Design review of the part built by this model. Coordinates are the model's own, in mm. A direction names the side the tool comes from. Round coordinates to 2 decimals unless told otherwise and drop trailing zeros. Write each loop counter-clockwise with the first axis right and the second up, starting at its lowest first coordinate (ties: lowest second). Pieces come first, ordered by that corner, then holes. Notation, with made-up numbers: (82, 54) -> (117, 54) arc R22 cw to (117, 82) -> close; hole circle Ø9 at (45.25, 7). An arc over 180 degrees is marked (long way). Write item = value, one per line. Start each with the question number.
Item 1: Add section C-C, the plane y = 1. State the section outline as (x, z) points.
Item 2: To check wall thickness, follow L1, parallel to X at y = -1.5, z = 14; L2, parallel to Y at x = 3.5, z = 6.5; L3, parallel to X at y = 3.25, z = 5. State the ranges of each line that lie inside material, in increasing order.
Item 3: Mouldability with a two-part tool opening along Z and no side actions: class faces 5 (the flat face through (-11, -2.6, 0)), 6 (the flat face through (-0.2, 0.4, 24.13)), 7 (the flat face through (-0.1, 1.5, -24.6)), 8 (the flat face through (0, 3, -19.13)) as released by +Z, released by -Z, zero draft, split by the parting line, or undercut.
Item 4: Add section B-B, the plane x = 5.25. State the section outline as (y, z) points, then the cut area to 3 significant figures.
Item 5: Add section A-A, the plane z = -7. State the section outline as (x, y) points, then the cut area to 3 significant figures.
Item 6: Machinability: for faces 1 (the flat face through (-0.2, 0.4, -24.13)), 2 (the flat face through (0, 4.1, -22)), 3 (the flat face through (7.5, 3, 8)), 4 (the flat face through (0, 0, 0)), which of the approach directions +Z, -Z, +X, -X, +Y, -Y give a long, thin tool a straight path to every point of the face, cutting with its end or side? Answer none if there is none.
Item 7: For pin 1 Ø1 at (x, z) = (9, 11.5) entering from -Y; pin 2 Ø1.3 at (y, z) = (3, -22) entering from -X; pin 3 Ø6 at (x, y) = (8.5, -1) entering from -Z, all flat-tipped, find the tip position at first contact; note any pin that passes through.
Item 8: Add section D-D, the plane y = -7. State the section outline as (x, z) points.
from build123d import *

# Parameters (mm, degrees)
SKETCH1_W           = 25.4
SKETCH1_H           = 48.26
BOSS_EXTRUDE1_DEPTH = 1.5
SKETCH2_W           = 15
SKETCH2_H           = 15
BOSS_EXTRUDE2_DEPTH = 3
SKETCH3_W           = 8
SKETCH3_H           = 6
BOSS_EXTRUDE3_DEPTH = 2.6
SKETCH4_W           = 2.54
SKETCH4_H           = 48.26
BOSS_EXTRUDE4_DEPTH = 2.6
SKETCH5_R           = 0.35
BOSS_EXTRUDE5_DEPTH = 5.9


with BuildPart() as part:
    # Sketch1 → Boss-Extrude1 (new body)
    with BuildSketch(Plane(origin=(0, 0, 0), x_dir=(1, 0, 0), z_dir=(0, 1, 0))):
        Rectangle(SKETCH1_W, SKETCH1_H)
    extrude(amount=BOSS_EXTRUDE1_DEPTH)

    # Sketch2 → Boss-Extrude2 (add)
    with BuildSketch(Plane(origin=(0, 1.5, 0), x_dir=(1, 0, 0), z_dir=(0, 1, 0))):
        with Locations((0, -7.5)):
            Rectangle(SKETCH2_W, SKETCH2_H)
    extrude(amount=BOSS_EXTRUDE2_DEPTH)

    # Sketch3 → Boss-Extrude3 (add)
    with BuildSketch(Plane(origin=(0, 1.5, 0), x_dir=(1, 0, 0), z_dir=(0, 1, 0))):
        with Locations((0, 22.13)):
            Rectangle(SKETCH3_W, SKETCH3_H)
    extrude(amount=BOSS_EXTRUDE3_DEPTH)

    # Sketch4 → Boss-Extrude4 (add)
    with BuildSketch(Plane.XZ):
        with Locations((-11.43, 0)):
            Rectangle(SKETCH4_W, SKETCH4_H)
        with Locations((11.43, 0)):
            Rectangle(SKETCH4_W, SKETCH4_H)
    extrude(amount=BOSS_EXTRUDE4_DEPTH)

    # Sketch5 → Boss-Extrude5 (add)
    with BuildSketch(Plane.XZ.offset(2.6)):
        with Locations(Location((11.43, -22.86, 0), (0, 0, 90))):
            Circle(SKETCH5_R)
        with Locations(Location((-11.43, -22.86, 0), (0, 0, 90))):
            Circle(SKETCH5_R)
        with Locations(Location((-11.43, 22.86, 0), (0, 0, 90))):
            Circle(SKETCH5_R)
        with Locations(Location((11.43, 22.86, 0), (0, 0, 90))):
            Circle(SKETCH5_R)
    extrude(amount=BOSS_EXTRUDE5_DEPTH)


solid = part.part
Result set:
q1.outline = (-12.7, -24.13) -> (12.7, -24.13) -> (12.7, 24.13) -> (-12.7, 24.13) -> close
q2.L1 = -12.7 to -10.16, 10.16 to 12.7
q2.L2 = 0 to 4.5
q2.L3 = -7.5 to 7.5
q3.face_5 = undercut
q3.face_6 = released by +Z
q3.face_7 = zero draft
q3.face_8 = undercut
q4.outline = (0, -24.13) -> (1.5, -24.13) -> (1.5, 0) -> (4.5, 0) -> (4.5, 15) -> (1.5, 15) -> (1.5, 24.13) -> (0, 24.13) -> close
q4.area = 117 mm²
q5.outline = (-12.7, -2.6) -> (-10.16, -2.6) -> (-10.16, 0) -> (10.16, 0) -> (10.16, -2.6) -> (12.7, -2.6) -> (12.7, 1.5) -> (-12.7, 1.5) -> close
q5.area = 51.3 mm²
q6.face_1 = -Z, +X, -X, -Y
q6.face_2 = -Z, +X, -X, +Y
q6.face_3 = +Z, -Z, +X, +Y
q6.face_4 = +Z, -Z, -Y
q7.pin_1 = 0
q7.pin_2 = -4
q7.pin_3 = -24.13
q8.outline = circle Ø0.7 at (-11.43, -22.86); circle Ø0.7 at (-11.43, 22.86); circle Ø0.7 at (11.43, -22.86); circle Ø0.7 at (11.43, 22.86)
